from build123d import *

# Parameters (mm, degrees)
F2_R           = 42.8625
F2_R_2         = 19.05
F3_DEPTH       = 12.7
F4_R           = 42.8625
F4_R_2         = 20.193
F5_DEPTH       = 12.7
F7_DEPTH       = 44.451
F9_D           = 6.3
F9_CBORE_D     = 11.25
F9_CBORE_DEPTH = 6


with BuildPart() as f1:
    # F0 (on Front) → F1 (revolve)
    with BuildSketch(Plane.XZ):
        with BuildLine():
            Line((-28.575, 69.85), (-28.575, 4.7625))
            Line((-28.575, 4.7625), (28.575, 4.7625))
            Line((28.575, 4.7625), (28.575, 69.85))
            ThreePointArc((28.575, 69.85), (21.1355122421, 87.8105122421), (3.175, 95.25))
            Line((3.175, 95.25), (-3.175, 95.25))
            ThreePointArc((-3.175, 95.25), (-21.1355122421, 87.8105122421), (-28.575, 69.85))
        make_face()
    revolve(axis=Axis((19.5088337422, 0, 0), (1, 0, 0)))

    # F2 (on face) → F3 (cut)
    with BuildSketch(Plane.YZ.offset(28.575)):
        Circle(F2_R)
        Circle(F2_R_2, mode=Mode.SUBTRACT)
    extrude(amount=-F3_DEPTH, mode=Mode.SUBTRACT)

    # F4 (on face) → F5 (cut)
    with BuildSketch(Plane(origin=(-28.575, 0, 0), x_dir=(0, -1, 0), z_dir=(-1, 0, 0))):
        Circle(F4_R)
        Circle(F4_R_2, mode=Mode.SUBTRACT)
    extrude(amount=-F5_DEPTH, mode=Mode.SUBTRACT)

    # F6 (on face) → F7 (cut, through all)
    with BuildSketch(Plane(origin=(-15.875, 0, 0), x_dir=(0, -1, 0), z_dir=(-1, 0, 0))):
        with BuildLine():
            ThreePointArc((-18.7203690505, -10.755272317), (-21.59, 0), (-18.7203690505, 10.755272317))
            ThreePointArc((-18.7203690505, 10.755272317), (-17.7738085484, 15.553880974), (-19.9394044545, 19.9394044545))
            Line((-19.9394044545, 19.9394044545), (-22.7184506514, 22.7184506514))
            ThreePointArc((-22.7184506514, 22.7184506514), (-28.9918287657, 24.8987035276), (-34.5927437834, 21.3295962815))
            ThreePointArc((-34.5927437834, 21.3295962815), (-40.64, 0), (-34.5927437834, -21.3295962815))
            ThreePointArc((-34.5927437834, -21.3295962815), (-28.9918287657, -24.8987035276), (-22.7184506514, -22.7184506514))
            Line((-22.7184506514, -22.7184506514), (-19.9394044545, -19.9394044545))
            ThreePointArc((-19.9394044545, -19.9394044545), (-17.7738085484, -15.553880974), (-18.7203690505, -10.755272317))
        make_face()
        with BuildLine():
            ThreePointArc((-8.315530073, -31.0339807244), (-7.0669953933, -37.5570119771), (-1.1756003406, -40.6229930438))
            ThreePointArc((-1.1756003406, -40.6229930438), (20.32, -35.1952724098), (35.768344124, -19.2933967623))
            ThreePointArc((35.768344124, -19.2933967623), (36.058824159, -12.6583084495), (31.0339807244, -8.315530073))
            Line((31.0339807244, -8.315530073), (27.2377330212, -7.2983285667))
            ThreePointArc((27.2377330212, -7.2983285667), (22.3569603251, -7.615629238), (18.6745235764, -10.8346790074))
            ThreePointArc((18.6745235764, -10.8346790074), (10.795, -18.6974884677), (0.0458454741, -21.5899513245))
            ThreePointArc((0.0458454741, -21.5899513245), (-4.5831517767, -23.1695102119), (-7.2983285667, -27.2377330212))
            Line((-7.2983285667, -27.2377330212), (-8.315530073, -31.0339807244))
        make_face()
        with BuildLine():
            ThreePointArc((31.0339807244, 8.315530073), (36.058824159, 12.6583084495), (35.768344124, 19.2933967623))
            ThreePointArc((35.768344124, 19.2933967623), (20.32, 35.1952724098), (-1.1756003406, 40.6229930438))
            ThreePointArc((-1.1756003406, 40.6229930438), (-7.0669953933, 37.5570119771), (-8.315530073, 31.0339807244))
            Line((-8.315530073, 31.0339807244), (-7.2983285667, 27.2377330212))
            ThreePointArc((-7.2983285667, 27.2377330212), (-4.5831517767, 23.1695102119), (0.0458454741, 21.5899513245))
            ThreePointArc((0.0458454741, 21.5899513245), (10.795, 18.6974884677), (18.6745235764, 10.8346790074))
            ThreePointArc((18.6745235764, 10.8346790074), (22.3569603251, 7.615629238), (27.2377330212, 7.2983285667))
            Line((27.2377330212, 7.2983285667), (31.0339807244, 8.315530073))
        make_face()
    extrude(amount=-F7_DEPTH, mode=Mode.SUBTRACT)

    # F9 (through all)
    with Locations(Plane.YZ.offset(15.875)):
        with Locations((14.097, -24.4167202343), (14.097, 24.4167202343), (-28.194, 0)):
            CounterBoreHole(F9_D / 2, F9_CBORE_D / 2, F9_CBORE_DEPTH)


solid = f1.part
The listing builds one solid part. Answer for the finished solid, in the listing's coordinates (mm). A direction names the side the tool comes from. Give positions to 0.01 mm unless a question says otherwise; leave off trailing zeros. One line per item, written item: value. Start each with the question number.
1) A tool of negligible diameter and unlimited length cuts with its end or side. For faces 4 (the face through (12.92, 17.12, 29.16)), 5 (the face through (-15.875, 6.6, 19.3)), 6 (the face through (-0.222, -22.293, 7.643)), from which of +Z, -Z, +X, -X, +Y, -Y can it reach the whole face along a straight path? Write none if from no direction.
2) A cutting plane is placed at A-A on x = 23. State how many separate pieces and enclosed holes the cut face has, then the cut area to 3 significant figures.
3) Given pin 1 Ø4 at (x, y) = (17, 43) entering from +Z; pin 2 Ø4 at (x, y) = (-17.5, -58) entering from -Z; pin 3 Ø12.5 at (y, z) = (15, -21.5) entering from +X (3 decimals), each flat-ended and moving along its own axis, determine where each tip first touches the part or whether it passes through.
4) Find the intervals of material crossed by L1, parallel to Z at x = -2, y = 13.5; L2, parallel to Z at x = 21.5, y = 0; L3, parallel to Z at x = 6, y = -34, in increasing order.
5) The mould has two halves that part along Y. Classify faces 1 (the face through (-0.22, -20.59, 35.04)), 2 (the face through (-22.314, 4.377, -19.713)), 3 (the face through (28.575, 30, 32)): released by +Y, released by -Y, zero draft, split by the parting line, or undercut.
Answer sheet:
1. face 4: +X
1. face 5: -X
1. face 6: +X, -X
2. separate pieces: 2
2. enclosed holes: 2
2. area: 18,400 mm2
3. pin 1: stops at z = 82.09
3. pin 2: stops at z = -72.19
3. pin 3: stops at x = 15.875
4. L1: z = -94.29 to -27.51, -21.32 to 21.32, 27.51 to 94.29
4. L2: z = -87.44 to -42.86, -19.05 to -4.76, 4.76 to 19.05, 42.86 to 87.44
4. L3: z = -88.81 to -22.26, -9.87 to 9.87, 22.26 to 88.81
5. face 1: undercut
5. face 2: undercut
5. face 3: zero draft
